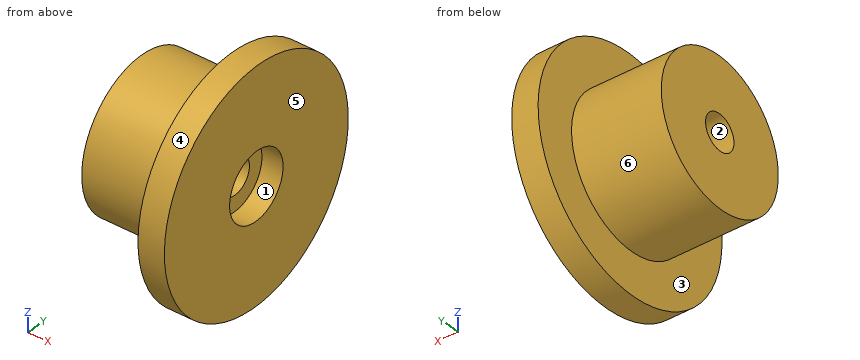
from build123d import *


with BuildPart() as part:
    # Sketch1 → Pin (revolve)
    with BuildSketch(Plane.XY, mode=Mode.PRIVATE) as pin_sk:
        Polygon((0, 1.7), (0, 7), (8.5, 7), (8.5, 11), (11, 11), (11, 3.2), (9, 3.2), (9, 1.7), align=None)
    revolve(pin_sk.sketch.rotate(Axis((-5, 0, 0), (1, 0, 0)), 90), axis=Axis((-5, 0, 0), (1, 0, 0)))


solid = part.part
Build history of the part. All positions in model axes, mm. Face numbers are marked on the shaded views. A direction names the side the tool comes from. Round coordinates to 2 decimals unless told otherwise and drop trailing zeros. Write each loop counter-clockwise with the first axis right and the second up, starting at its lowest first coordinate (ties: lowest second). Pieces come first, ordered by that corner, then holes. Notation, with made-up numbers: (-35.75, 14) -> (6.25, 14) arc R34 cw to (6.25, 44) -> close; hole circle Ø2 at (52, 13). An arc over 180 degrees is marked (long way). Write item = value, one per line.
(1) Band-saw the part on D-D (z = -5.25). Give the cut face in (x, y).
Answer:
outline = (0, -4.63) -> (8.5, -4.63) -> (8.5, -9.67) -> (11, -9.67) -> (11, 9.67) -> (8.5, 9.67) -> (8.5, 4.63) -> (0, 4.63) -> close
(2) Band-saw the part on A-A (y = 0). Give the cut face in (x, z), then the cut area to 3 significant figures.
Answer:
outline = (0, -7) -> (8.5, -7) -> (8.5, -11) -> (11, -11) -> (11, -3.2) -> (9, -3.2) -> (9, -1.7) -> (0, -1.7) -> close; (0, 1.7) -> (9, 1.7) -> (9, 3.2) -> (11, 3.2) -> (11, 11) -> (8.5, 11) -> (8.5, 7) -> (0, 7) -> close
area = 131 mm2
(3) Tool access for the marked faces 5 and 6: list every direction of +Z, -Z, +X, -X, +Y, -Y with a clear straight run to the whole face (end or side of a thin tool).
Answer:
face_5 = +Z, -Z, +X, +Y, -Y
face_6 = -X
(4) Two-plate mould, pull along Z, no slides. Class the marked faces 1, 2, 3 and 4: pulls with the +Z half, pulls with the -Z half, needs draft (parallel to the pull), parting line crosses it, or undercut.
Answer:
face_1 = undercut
face_2 = undercut
face_3 = needs draft
face_4 = parting line crosses it
(5) Probe L1, parallel to Y at x = 9.95, z = 0; L2, parallel to Y at x = 3.25, z = 0; L3, parallel to X at y = 10, z = -4. List the from-to ranges inside material, lowest first.
Answer:
L1 = -11 to -3.2, 3.2 to 11
L2 = -7 to -1.7, 1.7 to 7
L3 = 8.5 to 11
(6) Flat gauge pins, fed straight in: pin 1 (4 mm diameter, centred on x = 3.5, z = 0.5, fed in from +Y); pin 2 (4 mm diameter, centred on y = 0, z = 0, fed in from +X). Where does each tip first touch, or does it go through?
Answer:
pin_1 = 7
pin_2 = 9
(7) Band-saw the part on C-C (x = 10). Give the cut face in (y, z).
Answer:
outline = circle Ø22 at (0, 0); hole circle Ø6.4 at (0, 0)
